Geometry check sheet. Reference: the model listing, model coordinates, mm. Round coordinates to 2 decimals unless told otherwise and drop trailing zeros. Write each loop counter-clockwise with the first axis right and the second up, starting at its lowest first coordinate (ties: lowest second). Pieces come first, ordered by that corner, then holes. Notation, with made-up numbers: M -31,-3.5 L 18,-3.5 A22 cw 18,27.5 Z; hole C 44,65.5 d8. An arc over 180 degrees is marked long. Put each result on its own line as item: value. Start each with the question number.
(1) Material ranges on probe 1 along Y at (x, z) = (-21, 0.35); probe 2 along X at (y, z) = (630, 1.25), recorded low to high.
(2) Section check B-B on z = 0.65. Record the cut outline in (x, y).
(3) Section check A-A on x = 20. Record the cut outline in (y, z), then the cut area to 3 significant figures.
Solid Edge part; units mm, degrees
sketch "Sketch1" plane through (0, 0, 0) normal (0, 0, 1) x (1, 0, 0)
  line L0 (350, 750) -> (-350, 750)
  line L1 (-350, 750) -> (-350, -750)
  line L2 (-350, -750) -> (350, -750)
  line L3 (350, -750) -> (350, 750)
extrude "Protrusion1" add sketch "Sketch1" along normal blind 2
sketch "Sketch2" plane through (0, 0, 2) normal (0, 0, 1) x (1, 0, 0)
  line L0 (94, 516) -> (94, 650)
  line L1 (94, 650) -> (-94, 650)
  line L2 (-94, 650) -> (-94, 516)
  line L3 (-94, 516) -> (94, 516)
extrude "ExtrudedCutout_1" cut sketch "Sketch2" against normal blind 269.0392
properties material "Aluminum, 1060"
Answers follow:
1. probe 1: y = -750 to 516, 650 to 750
1. probe 2: x = -350 to -94, 94 to 350
2. outline: M -350,-750 L 350,-750 L 350,750 L -350,750 Z; hole M -94,516 L 94,516 L 94,650 L -94,650 Z
3. outline: M -750,0 L 516,0 L 516,2 L -750,2 Z; M 650,0 L 750,0 L 750,2 L 650,2 Z
3. area: 2,730 mm^2
